from build123d import *

# Parameters (mm, degrees)
F0_R     = 6
F1_DEPTH = 2.1
F2_R     = 6
F2_R_2   = 4
F3_DEPTH = 80
F4_R     = 6
F5_DEPTH = 0.5
F6_R     = 6
F7_DEPTH = 1


# Not quite as in the source:
# - after a boolean that leaves OpenCascade's solid faulty, fix() repairs it


with BuildPart() as f1:
    # F0 (on Top) → F1 (new body)
    with BuildSketch(Plane.XY):
        Circle(F0_R)
    extrude(amount=F1_DEPTH)

    # F2 (on face) → F3 (join)
    with BuildSketch(Plane.XY.offset(2.1)):
        Circle(F2_R)
        Circle(F2_R_2, mode=Mode.SUBTRACT)
    extrude(amount=F3_DEPTH)

    # F4 (on face) → F5 (join)
    with BuildSketch(Plane.XY.offset(82.1)):
        Circle(F4_R)
        with BuildLine():
            Line((0, 4), (0, 4.5))
            ThreePointArc((0, 4.5), (3.1819805153, 3.1819805153), (4.5, 0))
            Line((4.5, 0), (4, 0))
            ThreePointArc((4, 0), (2.8284271247, -2.8284271247), (0, -4))
            Line((0, -4), (0, -4.5))
            ThreePointArc((0, -4.5), (-3.1819805153, -3.1819805153), (-4.5, 0))
            Line((-4.5, 0), (-4, 0))
            ThreePointArc((-4, 0), (-2.8284271247, 2.8284271247), (0, 4))
        make_face(mode=Mode.SUBTRACT)
    extrude(amount=F5_DEPTH)

    add(f1.part.fix(), mode=Mode.REPLACE)

    # F6 (on face) → F7 (join)
    with BuildSketch(Plane.XY.offset(82.6)):
        Circle(F6_R)
        with BuildLine():
            ThreePointArc((-4, 0), (-2.8284271247, 2.8284271247), (0, 4))
            Line((0, 4), (0, 4.5))
            ThreePointArc((0, 4.5), (3.1819805153, 3.1819805153), (4.5, 0))
            Line((4.5, 0), (4, 0))
            ThreePointArc((4, 0), (2.8284271247, -2.8284271247), (0, -4))
            Line((0, -4), (0, -4.5))
            ThreePointArc((0, -4.5), (-0.2759966411, -4.4915282315), (-0.5509540913, -4.466144824))
            ThreePointArc((-0.5509540913, -4.466144824), (-3.1806256543, -3.1833347997), (-4.4656741218, -0.554756377))
            ThreePointArc((-4.4656741218, -0.554756377), (-4.4914103324, -0.2779086647), (-4.5, 0))
            Line((-4.5, 0), (-4, 0))
        make_face(mode=Mode.SUBTRACT)
        with BuildLine():
            ThreePointArc((-0.5509540913, -3.9618745045), (-2.8432495074, -2.813526655), (-3.9674454323, -0.5092904299))
            Line((-3.9674454323, -0.5092904299), (-4.4656741218, -0.554756377))
            ThreePointArc((-4.4656741218, -0.554756377), (-3.1806256543, -3.1833347997), (-0.5509540913, -4.466144824))
            Line((-0.5509540913, -4.466144824), (-0.5509540913, -3.9618745045))
        make_face()
    extrude(amount=F7_DEPTH)


solid = f1.part
Input: part model. Units: mm. Frame: model coordinates. A direction names the side the tool comes from. Round coordinates to 2 decimals unless told otherwise and drop trailing zeros. Order: outer loops, then holes, each group sorted by start corner. A loop starts at its lowest first (then second) coordinate and runs counter-clockwise, first axis right, second up. Notation, with made-up numbers: (10, -32.5) - (19, -32.5) arc R21 cw to (19, -8.5) - close; hole circle Ø2 at (44.5, -14.75). An arc over 180 degrees is marked (long way). Use a Markdown table: item, result.
1. Section C-C on y = -2.5. Return the cut outline in (x, z), then the cut area to 3 significant figures.
Evaluation:
| item | result |
|---|---|
| outline | (-5.45, 0) - (5.45, 0) - (5.45, 83.6) - (3.12, 83.6) - (3.12, 2.1) - (-3.12, 2.1) - (-3.12, 82.1) - (-3.74, 82.1) - (-3.74, 82.6) - (-3.12, 82.6) - (-3.12, 83.6) - (-5.45, 83.6) - close |
| area | 403 mm^2 |
2. Section D-D on x = -1.25. Return the cut outline in (y, z).
Evaluation:
| item | result |
|---|---|
| outline | (-5.87, 0) - (5.87, 0) - (5.87, 83.6) - (3.8, 83.6) - (3.8, 2.1) - (-3.8, 2.1) - (-3.8, 82.1) - (-4.32, 82.1) - (-4.32, 82.6) - (-3.8, 82.6) - (-3.8, 83.6) - (-5.87, 83.6) - close |
3. Section A-A on x = 3.25. Return the cut outline in (y, z).
Evaluation:
| item | result |
|---|---|
| outline | (-5.04, 0) - (5.04, 0) - (5.04, 83.6) - (3.11, 83.6) - (3.11, 82.1) - (2.33, 82.1) - (2.33, 2.1) - (-2.33, 2.1) - (-2.33, 83.6) - (-5.04, 83.6) - close |
4. Material intervals for probe 1 along Y at (x, z) = (0.25, 38); probe 2 along X at (y, z) = (-3.25, 7); probe 3 along Y at (x, z) = (-1.75, 45.5), sorted ascending.
Evaluation:
| item | result |
|---|---|
| probe 1 | -5.99 to -3.99, 3.99 to 5.99 |
| probe 2 | -5.04 to -2.33, 2.33 to 5.04 |
| probe 3 | -5.74 to -3.6, 3.6 to 5.74 |
5. Mould query, pull axis Z, two halves, no side actions, for faces 1 (the face through (-3, -3, 82.1)), 2 (the face through (0, 0, 0)), 3 (the face through (3.147, 3.217, 82.84)). Classes: +Z half, -Z half, draft (parallel to the pull), parting line (faces both ways), or undercut.
Evaluation:
| item | result |
|---|---|
| face 1 | undercut |
| face 2 | -Z half |
| face 3 | draft |
6. Access query for faces 4 (the face through (3, 3, 82.1)), 5 (the face through (-3, -3, 82.6)), 6 (the face through (-1.42, -3.92, 83.6)). Directions: +Z, -Z, +X, -X, +Y, -Y. A direction counts if a zero-diameter tool reaches every point of the face in a straight line with its end or side. Return the directions, or none.
Evaluation:
| item | result |
|---|---|
| face 4 | +Z |
| face 5 | none |
| face 6 | +Z, +X, -X, +Y, -Y |
7. First-contact query: pin 1 (0.6 mm diameter, centred on x = 4.5, z = 82.5, fed in from +Y); pin 2 (5 mm diameter, centred on x = -3.5, z = 33, fed in from +Y); pin 3 (1.3 mm diameter, centred on x = 2.5, y = 2, fed in from +Z). Flat tips, straight axial feed; report the tip coordinate or a pass-through.
Evaluation:
| item | result |
|---|---|
| pin 1 | y = 4.28 |
| pin 2 | y = 5.92 |
| pin 3 | z = 2.1 |
8. Section B-B on z = 33. Return the cut outline in (x, y).
Evaluation:
| item | result |
|---|---|
| outline | circle Ø12 at (0, 0); hole circle Ø8 at (0, 0) |
